```python
from build123d import *

# Parameters (mm, degrees)
SKETCH2_R               = 17.5
SKETCH2_R_2             = 15.9125
BOSS_EXTRUDE1_DEPTH     = 540
SKETCH6_W               = 2.75
SKETCH6_H               = 17.5
SKETCH7_R               = 17.5
SKETCH7_R_2             = 15.9125
BOSS_EXTRUDE2_DEPTH     = 130
SKETCH13_R              = 17.5
SKETCH13_R_2            = 15.9125
BOSS_EXTRUDE4_DEPTH     = 59.5
SKETCH12_R              = 2.75
CUT_EXTRUDE4_DEPTH      = 18.5000001
CUT_EXTRUDE4_DEPTH_BACK = 18.5000001
SKETCH14_R              = 2.5
CUT_EXTRUDE5_DEPTH      = 18.5000001
CUT_EXTRUDE5_DEPTH_BACK = 18.5000001
SKETCH15_R              = 2.5
CUT_EXTRUDE6_DEPTH      = 18.5000001
CUT_EXTRUDE6_DEPTH_BACK = 18.5000001


with BuildPart() as part:
    # Sketch2 → Boss-Extrude1 (new body, symmetric)
    with BuildSketch(Plane.XY):
        Circle(SKETCH2_R)
        Circle(SKETCH2_R_2, mode=Mode.SUBTRACT)
    extrude(amount=BOSS_EXTRUDE1_DEPTH, both=True)

    # Sketch6 → M5 Clearance Hole1 (revolve, cut)
    with BuildSketch(Plane(origin=(0, 0, -445), x_dir=(0, 0, -1), z_dir=(1, 0, 0))):
        with Locations((1.375, 8.75)):
            Rectangle(SKETCH6_W, SKETCH6_H)
    m5_clearance_hole1 = revolve(axis=Axis((0, -6.35, -445), (0, 1, 0)), mode=Mode.SUBTRACT)

    # Mirror1: M5 Clearance Hole1 across plane
    add(m5_clearance_hole1.mirror(Plane.ZX), mode=Mode.SUBTRACT)

    # Sketch7 → Boss-Extrude2 (add)
    with BuildSketch(Plane.XY.offset(540)):
        Circle(SKETCH7_R)
        Circle(SKETCH7_R_2, mode=Mode.SUBTRACT)
    extrude(amount=BOSS_EXTRUDE2_DEPTH)

    # Sketch13 → Boss-Extrude4 (add)
    with BuildSketch(Plane.XY.offset(670)):
        Circle(SKETCH13_R)
        Circle(SKETCH13_R_2, mode=Mode.SUBTRACT)
    extrude(amount=BOSS_EXTRUDE4_DEPTH)

    # Sketch12 → Cut-Extrude4 (cut, two sides)
    with BuildSketch(Plane(origin=(0, 0, 0), x_dir=(1, 0, 0), z_dir=(0, 1, 0))) as cut_extrude4_sk:
        with Locations((0, -644.5)):
            Circle(SKETCH12_R)
    extrude(amount=CUT_EXTRUDE4_DEPTH, mode=Mode.SUBTRACT)
    extrude(cut_extrude4_sk.sketch, amount=-CUT_EXTRUDE4_DEPTH_BACK, mode=Mode.SUBTRACT)

    # Sketch14 → Cut-Extrude5 (cut, two sides)
    with BuildSketch(Plane(origin=(0, 0, 0), x_dir=(1, 0, 0), z_dir=(0, 1, 0))) as cut_extrude5_sk:
        with Locations((0, 515)):
            Circle(SKETCH14_R)
    extrude(amount=CUT_EXTRUDE5_DEPTH, mode=Mode.SUBTRACT)
    extrude(cut_extrude5_sk.sketch, amount=-CUT_EXTRUDE5_DEPTH_BACK, mode=Mode.SUBTRACT)

    # Sketch15 → Cut-Extrude6 (cut, two sides)
    with BuildSketch(Plane(origin=(0, 0, 0), x_dir=(0, 0, -1), z_dir=(1, 0, 0))) as cut_extrude6_sk:
        with Locations((-379.5, 0)):
            Circle(SKETCH15_R)
    extrude(amount=CUT_EXTRUDE6_DEPTH, mode=Mode.SUBTRACT)
    extrude(cut_extrude6_sk.sketch, amount=-CUT_EXTRUDE6_DEPTH_BACK, mode=Mode.SUBTRACT)


solid = part.part
```
Work out the finished part from the listing and answer in its coordinate system (mm). Coordinates: 2 decimals unless noted, no trailing zeros. Loops run counter-clockwise (first coordinate to the right, second up) from the corner with the lowest first, then second, coordinate; pieces in that order, holes last. Notation, with made-up numbers: (-2, -15.5) - (11, -15.5) arc R17 cw to (11, -4.5) - close; hole circle Ø7 at (77, 54). An arc over 180 degrees is marked (long way). Use a Markdown table: item, result.
Item 1: The mould has two halves that part along X. Classify faces 1 (the cylindrical face through (-2.071, 15.777, 85.864)), 2 (the cylindrical face through (-13.887, -10.648, 85.864)), 3 (the flat face through (8, -14, -540)): +X half, -X half, draft (parallel to the pull), parting line (faces both ways), or undercut.
Evaluation:
| item | result |
|---|---|
| face 1 | undercut |
| face 2 | parting line |
| face 3 | draft |
Item 2: Consider probe 1 along Z at (x, y) = (0, -16); probe 2 along Y at (x, z) = (-1, -362.5); probe 3 along X at (y, z) = (-2, 165.5). Determine where each line is inside the solid, lowest interval first. Write a range as from..to.
Evaluation:
| item | result |
|---|---|
| probe 1 | z = -540..-517.5, -512.5..-447.75, -442.25..641.75, 647.25..729.5 |
| probe 2 | y = -17.47..-15.88, 15.88..17.47 |
| probe 3 | x = -17.39..-15.79, 15.79..17.39 |
Item 3: Given pin 1 Ø1 at (y, z) = (3, -105) entering from -X; pin 2 Ø10 at (y, z) = (-8.5, 254) entering from -X; pin 3 Ø4 at (x, z) = (-12, 533.5) entering from +Y, each flat-ended and moving along its own axis, determine where each tip first touches the part or whether it passes through.
Evaluation:
| item | result |
|---|---|
| pin 1 | stops at x = -17.32 |
| pin 2 | stops at x = -17.15 |
| pin 3 | stops at y = 14.36 |
Item 4: Find section A-A, the plane z = -313.5. Determine the outline of the cut face in (x, y) (1 decimal).
Evaluation:
| item | result |
|---|---|
| outline | circle Ø35 at (0, 0); hole circle Ø31.8 at (0, 0) |
